from build123d import *

# Parameters (mm, degrees)
F0_W     = 457.2
F0_H     = 685.8
F1_DEPTH = 76.2
F3_START = -152.4
F3_DEPTH = 457.2
F4_R     = 25.4
F5_DEPTH = 50.8


with BuildPart() as f1:
    # F0 (on Front) → F1 (new body)
    with BuildSketch(Plane.XZ):
        with Locations((36.8095165998, 227.3958778115)):
            Rectangle(F0_W, F0_H)
    extrude(amount=F1_DEPTH)

    # F2 (on face) → F3 (cut)
    with BuildSketch(Plane.XY.offset(570.2958778115).offset(F3_START)):
        with BuildLine():
            Line((-156.9259542905, -76.2), (233.0776903711, -76.2))
            ThreePointArc((233.0776903711, -76.2), (38.0758680403, -5.6591071606), (-156.9259542905, -76.2))
        make_face()
    extrude(amount=-F3_DEPTH, mode=Mode.SUBTRACT)

    # F4 (on face) → F5 (join)
    with BuildSketch(Plane(origin=(0, 0, 417.8958778115), x_dir=(1, 0, 0), z_dir=(0, 0, -1))):
        with Locations((47.3616681993, 42.6765345037)):
            Circle(F4_R)
    extrude(amount=F5_DEPTH)


solid = f1.part
Work out the finished part from the listing and answer in its coordinate system (mm). A direction names the side the tool comes from. Give positions to 0.01 mm unless a question says otherwise; leave off trailing zeros. Write each loop counter-clockwise with the first axis right and the second up, starting at its lowest first coordinate (ties: lowest second). Pieces come first, ordered by that corner, then holes. Notation, with made-up numbers: (44, 0.25) - (71, 0.25) arc R27 cw to (71, 39.25) - close; hole circle Ø5 at (39, 21). An arc over 180 degrees is marked (long way). One line per item, written item: value. Start each with the question number.
1. For a pull along X with two mould halves and no side action, classify faces 3 (the cylindrical face through (44.06, -67.86, 392.85)), 4 (the flat face through (265.41, -38, 223)), 5 (the flat face through (34, 0, 232)) as +X half, -X half, draft (parallel to the pull), parting line (faces both ways), or undercut.
2. Given pin 1 (5 mm diameter, centred on x = 36, z = 323.5, fed in from -Y); pin 2 (10 mm diameter, centred on x = -105.5, z = 219, fed in from -Y), each flat-ended and moving along its own axis, determine where each tip first touches the part or whether it passes through.
3. Find section C-C (x = 56). Write down the section's boundary in (y, z).
4. Find section B-B (y = -55). Write down the section's boundary in (x, z), then the cut area to 3 significant figures.
5. Find section A-A (z = 381). Write down the section's boundary in (x, y).
6. For faces 1 (the flat face through (34, -76.2, 461)), 2 (the flat face through (47, -43, 367.096)), determine the directions among +Z, -Z, +X, -X, +Y, -Y from which every point of the face is accessible in a straight line to the end or side of a thin tool.
7. Find section D-D (z = -3.5). Write down the section's boundary in (x, y), then the cut area to 3 significant figures.
8. Consider probe 1 along Z at (x, y) = (88, -49); probe 2 along Z at (x, y) = (72, -45.5); probe 3 along X at (y, z) = (-35, 120.5). Determine where each line is inside the solid, lowest interval first.
Geometry results:
1. face 3: undercut
1. face 4: +X half
1. face 5: draft
2. pin 1: y = -5.69
2. pin 2: y = -44.32
3. outline: (-76.2, -115.5) - (0, -115.5) - (0, 570.3) - (-76.2, 570.3) - (-76.2, 417.9) - (-66.56, 417.9) - (-66.56, 367.1) - (-18.79, 367.1) - (-18.79, 417.9) - (-6.19, 417.9) - (-6.19, -39.3) - (-76.2, -39.3) - close
4. outline: (-191.79, -115.5) - (265.41, -115.5) - (265.41, 570.3) - (-191.79, 570.3) - close; hole (-128.19, -39.3) - (204.34, -39.3) - (204.34, 417.9) - (69.57, 417.9) - (69.57, 367.1) - (25.15, 367.1) - (25.15, 417.9) - (-128.19, 417.9) - close
4. area: 164,000 mm2
5. outline: (-191.79, -76.2) - (-156.93, -76.2) arc R304.8 cw to (233.08, -76.2) - (265.41, -76.2) - (265.41, 0) - (-191.79, 0) - close; circle Ø50.8 at (47.36, -42.68)
6. face 1: +Z, -Z, +X, -X, -Y
6. face 2: -Y
7. outline: (-191.79, -76.2) - (-156.93, -76.2) arc R304.8 cw to (233.08, -76.2) - (265.41, -76.2) - (265.41, 0) - (-191.79, 0) - close
7. area: 16,000 mm2
8. probe 1: -115.5 to -39.3, 417.9 to 570.3
8. probe 2: -115.5 to -39.3, 367.1 to 570.3
8. probe 3: -191.79 to -92.41, 168.56 to 265.41
